Geometry check sheet. Reference: the model listing, model coordinates, mm. Face numbers are marked on the shaded views. A direction names the side the tool comes from. Give positions to 0.01 mm unless a question says otherwise; leave off trailing zeros. Loops run counter-clockwise (first coordinate to the right, second up) from the corner with the lowest first, then second, coordinate; pieces in that order, holes last. Notation, with made-up numbers: (87.5, 86) -> (117.5, 86) arc R16 cw to (117.5, 92) -> close; hole circle Ø1 at (7, -21). An arc over 180 degrees is marked (long way). Answer as a JSON object with one key per item and string values.
Autodesk Inventor part; units mm, degrees
ref_plane "YZ Plane" through (0, 0, 0) normal (1, 0, 0) x (0, 1, 0)
ref_plane "XZ Plane" through (0, 0, 0) normal (0, 1, 0) x (-1, 0, 0)
ref_plane "XY Plane" through (0, 0, 0) normal (0, 0, 1) x (1, 0, 0)
sketch "Эскиз1" plane through (0, 0, 0) normal (0, 1, 0) x (-1, 0, 0)
  line L0 (-15.5, 20.5) -> (15.5, 20.5)
  line L1 (15.5, 20.5) -> (15.5, -20.5)
  line L2 (15.5, -20.5) -> (-15.5, -20.5)
  line L3 (-15.5, -20.5) -> (-15.5, 20.5)
  line L4 (-15.5, 20.5) -> (15.5, -20.5) construction
  line L5 (15.5, 20.5) -> (-15.5, -20.5) construction
  point P0 (0, 0)
  dimension "d0" = 41
  dimension "d1" = 31
extrude "Выдавливание1" add sketch "Эскиз1" along normal blind 1.5
sketch "Эскиз2" plane through (0, 1.5, 0) normal (0, 1, 0) x (1, 0, 0)
  line L0 (-1.5, -12.5) -> (5.5, -12.5)
  line L1 (5.5, -12.5) -> (5.5, -2.5)
  line L2 (5.5, -2.5) -> (-1.5, -2.5)
  line L3 (-1.5, -2.5) -> (-1.5, -12.5)
  line L4 (-1.5, -12.5) -> (5.5, -2.5) construction
  line L5 (5.5, -12.5) -> (-1.5, -2.5) construction
  line L6 (-2.5, 1.5) -> (5.5, 1.5)
  line L7 (5.5, 1.5) -> (5.5, 7.5)
  line L8 (5.5, 7.5) -> (-2.5, 7.5)
  line L9 (-2.5, 7.5) -> (-2.5, 1.5)
  line L10 (-2.5, 1.5) -> (5.5, 7.5) construction
  line L11 (5.5, 1.5) -> (-2.5, 7.5) construction
  line L12 (3.5, 10.5) -> (6.5, 10.5)
  line L13 (6.5, 10.5) -> (6.5, 14.5)
  line L14 (6.5, 14.5) -> (3.5, 14.5)
  line L15 (3.5, 14.5) -> (3.5, 10.5)
  line L16 (3.5, 10.5) -> (6.5, 14.5) construction
  line L17 (6.5, 10.5) -> (3.5, 14.5) construction
  line L18 (-3.5, 16.5) -> (-0.5, 16.5)
  line L19 (-0.5, 16.5) -> (-0.5, 12.5)
  line L20 (-0.5, 12.5) -> (-3.5, 12.5)
  line L21 (-3.5, 12.5) -> (-3.5, 16.5)
  line L22 (-3.5, 16.5) -> (-0.5, 12.5) construction
  line L23 (-0.5, 16.5) -> (-3.5, 12.5) construction
  line L24 (-8.5, 5.5) -> (-4.5, 5.5)
  line L25 (-4.5, 5.5) -> (-4.5, 1.5)
  line L26 (-4.5, 1.5) -> (-8.5, 1.5)
  line L27 (-8.5, 1.5) -> (-8.5, 5.5)
  line L28 (-8.5, 5.5) -> (-4.5, 1.5) construction
  line L29 (-4.5, 5.5) -> (-8.5, 1.5) construction
  line L30 (15.5, 20.5) -> (-15.5, 20.5)
  line L31 (15.5, -20.5) -> (15.5, 20.5)
  line L32 (-15.5, -20.5) -> (15.5, -20.5)
  point P0 (0, 0)
  point P1 (2, -7.5)
  point P2 (1.5, 4.5)
  point P3 (5, 12.5)
  point P4 (-2, 14.5)
  point P5 (-6.5, 3.5)
  dimension "d4" = 4
  dimension "d5" = 4
  dimension "d6" = 3
  dimension "d7" = 4
  dimension "d8" = 3
  dimension "d9" = 6
  dimension "d10" = 8
  dimension "d11" = 7
  dimension "d12" = 10
  dimension "d13" = 6
  dimension "d14" = 4
  dimension "d15" = 16
  dimension "d16" = 9
  dimension "d17" = 15
  dimension "d18" = 20
  dimension "d19" = 13
  dimension "d20" = 10
  dimension "d21" = 10
  dimension "d22" = 8
extrude "Выдавливание2" add sketch "Эскиз2" along normal blind 2
sketch "Эскиз3" plane through (0, 0, 0) normal (0, -1, 0) x (1, 0, 0)
  line L0 (-6.5, -9) -> (9.5, -9)
  line L1 (9.5, -9) -> (9.5, 9)
  line L2 (9.5, 9) -> (-6.5, 9)
  line L3 (-6.5, 9) -> (-6.5, -9)
  line L4 (-6.5, -9) -> (9.5, 9) construction
  line L5 (9.5, -9) -> (-6.5, 9) construction
  line L6 (15.5, 20.5) -> (15.5, -20.5)
  line L7 (-10.5, -4) -> (-6.5, -4)
  line L8 (-6.5, -4) -> (-6.5, 4)
  line L9 (-6.5, 4) -> (-10.5, 4)
  line L10 (-10.5, 4) -> (-10.5, -4)
  line L11 (-10.5, -4) -> (-6.5, 4) construction
  line L12 (-6.5, -4) -> (-10.5, 4) construction
  line L13 (-15.5, -20.5) -> (-15.5, 20.5)
  point P0 (0, 0)
  point P1 (1.5, 0)
  point P2 (1.5, 0)
  point P3 (-8.5, 0)
  point P4 (-8.5, 0)
  dimension "d25" = 16
  dimension "d26" = 18
  dimension "d27" = 6
  dimension "d28" = 8
  dimension "d29" = 4
  dimension "d30" = 5
extrude "Выдавливание3" add sketch "Эскиз3" along normal blind 5 contours L3 L2 L1 L0
sketch "Эскиз4" plane through (0, 0, 0) normal (0, -1, 0) x (1, 0, 0)
  line L0 (-6.5, 4) -> (-10.5, 4)
  line L1 (-10.5, 4) -> (-10.5, -4)
  line L2 (-10.5, -4) -> (-6.5, -4)
  line L3 (-6.5, -4) -> (-6.5, 4)
  line L4 (-6.5, 4) -> (-10.5, -4) construction
  line L5 (-10.5, 4) -> (-6.5, -4) construction
  line L6 (-15.5, -20.5) -> (-15.5, 20.5)
  point P0 (0, 0)
  point P1 (-8.5, 0)
  point P2 (-8.5, 0)
  dimension "d33" = 4
  dimension "d34" = 8
  dimension "d35" = 5
extrude "Выдавливание4" add sketch "Эскиз4" along normal blind 2
properties part number "РБАСУ" material "Пластик АБС"
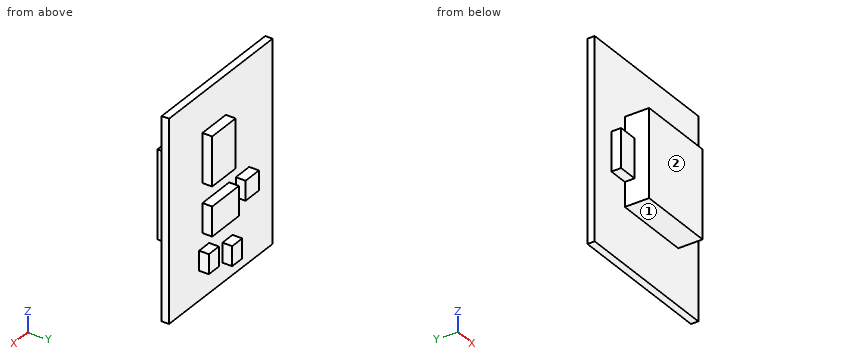
1) Section check A-A on y = 2.5. Record the cut outline in (x, z), plus the area to 3 significant figures.
Geometry check:
{"outline": "(-8.5, -5.5) -> (-4.5, -5.5) -> (-4.5, -1.5) -> (-8.5, -1.5) -> close; (-3.5, -16.5) -> (-0.5, -16.5) -> (-0.5, -12.5) -> (-3.5, -12.5) -> close; (-2.5, -7.5) -> (5.5, -7.5) -> (5.5, -1.5) -> (-2.5, -1.5) -> close; (-1.5, 2.5) -> (5.5, 2.5) -> (5.5, 12.5) -> (-1.5, 12.5) -> close; (3.5, -14.5) -> (6.5, -14.5) -> (6.5, -10.5) -> (3.5, -10.5) -> close", "area": "158 mm2"}
2) Material ranges on line 1 along Y through (x, z) = (9, 14); line 2 along Z through (x, y) = (7.5, -4); line 3 along Z through (x, y) = (3, 1.75), recorded low to high. Write a range as from..to.
Geometry check:
{"line 1": "y = 0..1.5", "line 2": "z = -9..9", "line 3": "z = -7.5..-1.5, 2.5..12.5"}
3) Depth check by flat-ended pin: P1, Ø1.6, axis at x = 3.5, y = 2.5, coming from the -Z side; P2, Ø1.6, axis at y = 2.5, z = -14, coming from the +X side; P3, Ø1.5, axis at x = 1, y = -3, coming from the +Z side. Enter the tip coordinate at first touch or a pass-through.
Geometry check:
{"P1": "stops at z = -14.5", "P2": "stops at x = 6.5", "P3": "stops at z = 9"}
4) Section check D-D on y = -1. Record the cut outline in (x, z), plus the area to 3 significant figures.
Geometry check:
{"outline": "(-10.5, -4) -> (-6.5, -4) -> (-6.5, -9) -> (9.5, -9) -> (9.5, 9) -> (-6.5, 9) -> (-6.5, 4) -> (-10.5, 4) -> close", "area": "320 mm2"}
5) Section check C-C on x = -7. Record the cut outline in (y, z), plus the area to 3 significant figures.
Geometry check:
{"outline": "(-2, -4) -> (0, -4) -> (0, -20.5) -> (1.5, -20.5) -> (1.5, -5.5) -> (3.5, -5.5) -> (3.5, -1.5) -> (1.5, -1.5) -> (1.5, 20.5) -> (0, 20.5) -> (0, 4) -> (-2, 4) -> close", "area": "85.5 mm2"}
6) Section check B-B on z = 0. Record the cut outline in (x, y), plus the area to 4 significant figures.
Geometry check:
{"outline": "(-15.5, 0) -> (-10.5, 0) -> (-10.5, -2) -> (-6.5, -2) -> (-6.5, -5) -> (9.5, -5) -> (9.5, 0) -> (15.5, 0) -> (15.5, 1.5) -> (-15.5, 1.5) -> close", "area": "134.5 mm2"}
7) Tool access check on the marked faces 1 and 2. Record the directions out of +Z, -Z, +X, -X, +Y, -Y that give a thin tool (end or side, any length) a straight path to the whole face; none if there is none.
Geometry check:
{"face 1": "-Z, +X, -X, -Y", "face 2": "+Z, -Z, +X, -X, -Y"}
